Build history of the part. All positions in model axes, mm. Face numbers are marked on the shaded views. A direction names the side the tool comes from. Round coordinates to 2 decimals unless told otherwise and drop trailing zeros. Write each loop counter-clockwise with the first axis right and the second up, starting at its lowest first coordinate (ties: lowest second). Pieces come first, ordered by that corner, then holes.
Item 1: 3-axis set-ups, long thin cutter, end or side, ignore diameter. For the marked faces 1, 2 and 3: which of +Z, -Z, +X, -X, +Y, -Y reach the whole face in a straight line?
Item 2: Drop flat-ended pins along their axis: pin 1 Ø2.5 at (x, z) = (-4, 74.1) entering from +Y; pin 2 Ø1.4 at (y, z) = (2, -8.5) entering from -X; pin 3 Ø10 at (x, z) = (-17, -17) entering from +Y; pin 4 Ø0.9 at (y, z) = (2, -11.5) entering from +X. Give the stop position or say it passes through.
Item 3: Band-saw the part on C-C, the plane x = -13.25. Write the cut outline in (y, z).
Item 4: Band-saw the part on A-A, the plane x = -26. Write the cut outline in (y, z), then the cut area to 3 significant figures.
Item 5: Band-saw the part on B-B, the plane z = 74.1. Write the cut outline in (x, y).
Item 6: Wall check: probe 1 along X at (y, z) = (3.9, 106); probe 2 along Z at (x, y) = (-26, 2.85); probe 3 along Z at (x, y) = (-5.25, 3.05). Give the ranges that are in metal, low to high.
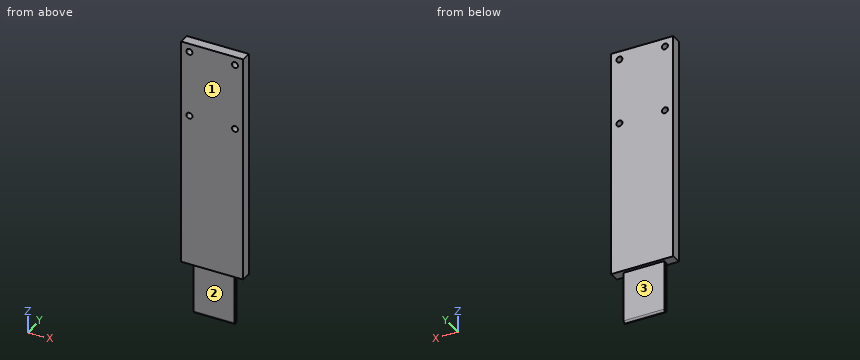
```python
from build123d import *

# Parameters (mm, degrees)
SKETCH_1_W          = 30
SKETCH_1_H          = 5
EXTRUDE_1_DEPTH     = 110
SKETCH_2_R          = 1.45
CUT_EXTRUDE_1_DEPTH = 60
SKETCH_4_W          = 19.6
SKETCH_4_H          = 1.8
EXTRUDE_2_DEPTH     = 25
FILLET_1_R          = 1


with BuildPart() as part:
    # 草图1 → 凸台-拉伸1 (new body)
    with BuildSketch(Plane.XY):
        with Locations((-15, 2.5)):
            Rectangle(SKETCH_1_W, SKETCH_1_H)
    extrude(amount=EXTRUDE_1_DEPTH)

    # 草图2 → 切除-拉伸1 (cut)
    with BuildSketch(Plane(origin=(0, 5, 0), x_dir=(1, 0, 0), z_dir=(0, 1, 0))):
        with Locations(Location((-26, -106, 0), (0, 0, 180))):
            Circle(SKETCH_2_R)
        with Locations(Location((-26, -74.1, 0), (0, 0, 180))):
            Circle(SKETCH_2_R)
        with Locations(Location((-4, -106, 0), (0, 0, 270))):
            Circle(SKETCH_2_R)
        with Locations(Location((-4, -74.1, 0), (0, 0, 270))):
            Circle(SKETCH_2_R)
    extrude(amount=-CUT_EXTRUDE_1_DEPTH, mode=Mode.SUBTRACT)

    # 草图4 → 凸台-拉伸2 (add)
    with BuildSketch(Plane(origin=(0, 0, 0), x_dir=(-1, 0, 0), z_dir=(0, 0, -1))):
        with Locations((15, 2.5)):
            Rectangle(SKETCH_4_W, SKETCH_4_H)
    extrude(amount=EXTRUDE_2_DEPTH)

    # 圆角1
    # the kernel refuses this fillet: 1 mm, written as the material it takes off along each edge
    with BuildSketch(Plane(origin=(-27.3, 1.6, -25), x_dir=(0, 0, 1), z_dir=(1, 0, 0)), Plane(origin=(-2.7, 3.4, -25), x_dir=(0, 0, 1), z_dir=(-1, 0, 0))) as fillet_1_piece_1:
        with BuildLine():
            CenterArc((FILLET_1_R, -FILLET_1_R), FILLET_1_R, 90, 90)
            Line((0, -FILLET_1_R), (0, 0))
            Line((0, 0), (FILLET_1_R, 0))
        make_face()
    extrude(amount=24.6, mode=Mode.SUBTRACT)


solid = part.part
```
Results:
1. face 1: +Z, -Z, +X, -X, -Y
1. face 2: -Z, +X, -X, -Y
1. face 3: -Z, +X, -X, +Y
2. pin 1: passes through
2. pin 2: stops at x = -24.8
2. pin 3: stops at y = 3.4
2. pin 4: stops at x = -5.2
3. outline: (0, 0) - (1.6, 0) - (1.6, -24) arc R1 ccw to (2.5, -24.99) arc R1 ccw to (3.4, -24) - (3.4, 0) - (5, 0) - (5, 110) - (0, 110) - close
4. outline: (0, 0) - (5, 0) - (5, 72.65) - (0, 72.65) - close; (0, 75.55) - (5, 75.55) - (5, 104.55) - (0, 104.55) - close; (0, 107.45) - (5, 107.45) - (5, 110) - (0, 110) - close
4. area: 521 mm2
5. outline: (-30, 0) - (-27.45, 0) - (-27.45, 5) - (-30, 5) - close; (-24.55, 0) - (-5.45, 0) - (-5.45, 5) - (-24.55, 5) - close; (-2.55, 0) - (0, 0) - (0, 5) - (-2.55, 5) - close
6. probe 1: x = -30 to -27.45, -24.55 to -5.45, -2.55 to 0
6. probe 2: z = 0 to 72.65, 75.55 to 104.55, 107.45 to 110
6. probe 3: z = -24.76 to 73.37, 74.83 to 105.27, 106.73 to 110
